```python
from build123d import *

# Parameters (mm, degrees)
F0_W          = 152.4
F0_H          = 6.35
F1_DEPTH      = 50.8
F3_DEPTH      = 76.2
F3_DEPTH_BACK = 25.4
F4_R          = 9.525
F5_DEPTH      = 25.155085


with BuildPart() as f1:
    # F0 (on Right) → F1 (new body)
    with BuildSketch(Plane.YZ):
        with Locations((12.980076, 9.279085)):
            Rectangle(F0_W, F0_H)
    extrude(amount=F1_DEPTH)

    # F2 (on Right) → F3 (join, two sides)
    with BuildSketch(Plane.YZ) as f3_sk:
        Polygon((-63.219924, -6.595915), (-63.219924, 12.454085), (-63.219924, 25.154085), (-69.569924, 25.154085), (-69.569924, -6.595915), align=None)
    extrude(amount=F3_DEPTH)
    extrude(f3_sk.sketch, amount=-F3_DEPTH_BACK)

    # F4 (on Top) → F5 (cut, through all)
    with BuildSketch(Plane.XY):
        with Locations((25.4, 70.130076)):
            Circle(F4_R)
    extrude(amount=F5_DEPTH, mode=Mode.SUBTRACT)


solid = f1.part
```
Build history of the part. All positions in model axes, mm. A direction names the side the tool comes from. Give positions to 0.01 mm unless a question says otherwise; leave off trailing zeros. Order: outer loops, then holes, each group sorted by start corner. A loop starts at its lowest first (then second) coordinate and runs counter-clockwise, first axis right, second up. Notation, with made-up numbers: M 37,-1 L 68,-1 A29 cw 68,31 Z; hole C 51,60 d10. An arc over 180 degrees is marked long. Write item = value, one per line. Start each with the question number.
(1) Slice it at D-D on y = 19.5. Write the cut outline in (x, z).
(2) Probe L1, parallel to Y at x = 25.4, z = 9.5; L2, parallel to Y at x = 25, z = 9; L3, parallel to X at y = 24, z = 11. List the from-to ranges inside material, lowest first. Write a range as [from, to].
(3) Two-plate mould, pull along Y, no slides. Class faces 1 (the flat face through (26, -66, 25.154)), 2 (the cylindrical face through (18.38, 76.57, 9.23)), 3 (the flat face through (25, 89.18, 9)): released by +Y, released by -Y, zero draft, split by the parting line, or undercut.
(4) Which spindle directions (+Z, -Z, +X, -X, +Y, -Y) get a long thin tool onto all of the face, cutting with end or side? Do faces 4 (the flat face through (0, 12, 9)), 5 (the flat face through (50.8, 12, 9)), 6 (the flat face through (25, 12, 6.104)). Say none if no direction does.
(5) Slice it at A-A on x = 25.4. Write the cut outline in (y, z).
(6) Pin check, flat tips, straight feed: pin 1 Ø7 at (y, z) = (-12, 10) entering from -X; pin 2 Ø5 at (y, z) = (49, 10.5) entering from +X; pin 3 Ø12 at (x, y) = (-5.5, 2.5) entering from -Z. Stop position of each tip, or through.
(7) Slice it at C-C on x = 12. Write the cut outline in (y, z), plus the area to 3 significant figures.
(8) Slice it at B-B on z = 9. Write the cut outline in (x, y) (3 decimals).
Responses:
q1.outline = M 0,6.1 L 50.8,6.1 L 50.8,12.45 L 0,12.45 Z
q2.L1 = [-69.57, 60.61], [79.66, 89.18]
q2.L2 = [-69.57, 60.61], [79.65, 89.18]
q2.L3 = [0, 50.8]
q3.face_1 = zero draft
q3.face_2 = undercut
q3.face_3 = released by +Y
q4.face_4 = +Z, -Z, -X, +Y
q4.face_5 = +Z, -Z, +X, +Y
q4.face_6 = -Z, +X, -X, +Y
q5.outline = M -69.57,-6.6 L -63.22,-6.6 L -63.22,6.1 L 60.61,6.1 L 60.61,12.45 L -63.22,12.45 L -63.22,25.15 L -69.57,25.15 Z; M 79.66,6.1 L 89.18,6.1 L 89.18,12.45 L 79.66,12.45 Z
q6.pin_1 = 0
q6.pin_2 = 50.8
q6.pin_3 = 6.1
q7.outline = M -69.57,-6.6 L -63.22,-6.6 L -63.22,6.1 L 89.18,6.1 L 89.18,12.45 L -63.22,12.45 L -63.22,25.15 L -69.57,25.15 Z
q7.area = 1,170 mm2
q8.outline = M -25.4,-69.57 L 76.2,-69.57 L 76.2,-63.22 L 50.8,-63.22 L 50.8,89.18 L 0,89.18 L 0,-63.22 L -25.4,-63.22 Z; hole C 25.4,70.13 d19.05
